Check sheet for the drawn part. Datum: minimum x, y, z corner. Units: mm. A direction names the side the tool comes from. Coordinates: 2 decimals unless noted, no trailing zeros. Order: outer loops, then holes, each group sorted by start corner. A loop starts at its lowest first (then second) coordinate and runs counter-clockwise, first axis right, second up. Notation, with made-up numbers: M 89.5,89 L 132.5,89 A23 cw 132.5,116 Z; hole C 40,-37.5 d10. An arc over 180 degrees is marked long. Return JSON: item names as keys, results as strings. Group by question number.
Q1. Mould release check, pull along Z, two halves, no side actions. Record for the marked faces 3, 4 and 5: pulls with the +Z half, pulls with the -Z half, needs draft (parallel to the pull), parting line crosses it, or undercut.
Q2. Access from +Z, -Z, +X, -X, +Y, -Y to the whole of each face (thin tool, end or side, straight path). Record for the marked faces 1 and 2.
Q3. Thickness scan on probe 1 along X at (y, z) = (2.1, 9) (1 decimal); probe 2 along X at (y, z) = (4.05, 8) (1 decimal); probe 3 along X at (y, z) = (0.45, 9.5). Record the ranges inside material, lowest first.
Q4. Section check C-C, the plane x = 2.25. Enter the section's corners in (y, z).
Q5. Section check B-B, the plane z = 9. Enter the section's corners in (x, y) (1 decimal).
Q6. Section check A-A, the plane x = 9. Enter the section's corners in (y, z) (1 decimal), then the cut area to 3 significant figures.
Q7. Section check D-D, the plane z = 2. Enter the section's corners in (x, y) (1 decimal).
Q8. Go/stop test with flat-tipped pins: pin 1 Ø1 at (y, z) = (1.5, 7) entering from -X; pin 2 Ø1.5 at (x, y) = (7, 3.5) entering from -Z; pin 3 Ø1 at (x, y) = (6.5, 2) entering from -Z (3 decimals). Record where each tip stops, or that it passes through.
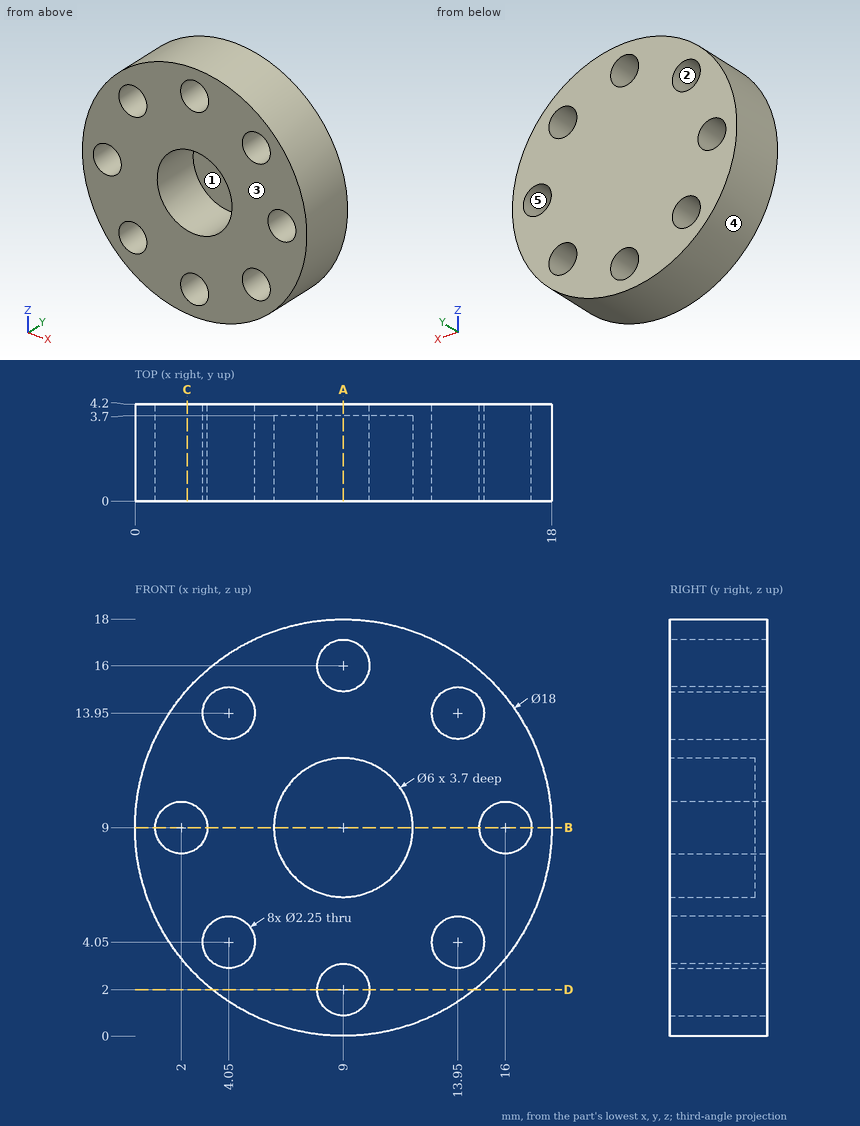
Numbers:
{
 "1": {"face 3": "needs draft", "face 4": "parting line crosses it", "face 5": "undercut"},
 "2": {"face 1": "-Y", "face 2": "+Y, -Y"},
 "3": {"probe 1": "x = 0 to 0.9, 3.1 to 6, 12 to 14.9, 17.1 to 18", "probe 2": "x = 0.1 to 1.5, 2.5 to 15.5, 16.5 to 17.9", "probe 3": "x = 0.01 to 0.99, 3.01 to 6.04, 11.96 to 14.99, 17.01 to 17.99"},
 "4": {"outline": "M 0,3.05 L 4.2,3.05 L 4.2,7.9 L 0,7.9 Z; M 0,10.1 L 4.2,10.1 L 4.2,14.95 L 0,14.95 Z"},
 "5": {"outline": "M 0,0 L 0.9,0 L 0.9,4.2 L 0,4.2 Z; M 3.1,0 L 6,0 L 6,3.7 L 12,3.7 L 12,0 L 14.9,0 L 14.9,4.2 L 3.1,4.2 Z; M 17.1,0 L 18,0 L 18,4.2 L 17.1,4.2 Z"},
 "6": {"outline": "M 0,0 L 4.2,0 L 4.2,0.9 L 0,0.9 Z; M 0,3.1 L 4.2,3.1 L 4.2,14.9 L 0,14.9 L 0,12 L 3.7,12 L 3.7,6 L 0,6 Z; M 0,17.1 L 4.2,17.1 L 4.2,18 L 0,18 Z", "area": "34.5 mm2"},
 "7": {"outline": "M 3.3,0 L 7.9,0 L 7.9,4.2 L 3.3,4.2 Z; M 10.1,0 L 14.7,0 L 14.7,4.2 L 10.1,4.2 Z"},
 "8": {"pin 1": "stops at x = 0.13", "pin 2": "stops at z = 0.09", "pin 3": "stops at z = 0.225"}
}
